Work out the finished part from the listing and answer in its coordinate system (mm). Round coordinates to 2 decimals unless told otherwise and drop trailing zeros. Write each loop counter-clockwise with the first axis right and the second up, starting at its lowest first coordinate (ties: lowest second). Pieces come first, ordered by that corner, then holes. Notation, with made-up numbers: M -16.75,-12.5 L -11.75,-12.5 A19 cw -11.75,-5.5 Z; hole C -15.5,45 d8. An arc over 180 degrees is marked long. One line per item, written item: value. Start each with the question number.
Q1. Find section B-B (x = 632). Write down the section's boundary in (y, z).
Q2. Find section A-A (y = 488.75). Write down the section's boundary in (x, z), and give its area (3 significant figures).
Q3. Consider probe 1 along X at (y, z) = (491.5, 1847); probe 2 along X at (y, z) = (486.5, 1922.5); probe 3 along Z at (x, y) = (610, 487.5). Determine where each line is inside the solid, lowest interval first.
Q4. Find section C-C (z = 1811). Write down the section's boundary in (x, y), and give its area (3 significant figures).
Q5. Given pin 1 Ø1 at (x, y) = (996.5, 487) entering from -Z; pin 2 Ø6.5 at (x, z) = (605.22, 1770.69) entering from +Y; pin 3 Ø2 at (y, z) = (486, 1840) entering from +X; pin 4 Ø6.5 at (x, z) = (979.33, 1620) entering from -Y, each flat-ended and moving along its own axis, determine where each tip first touches the part or whether it passes through.
from build123d import *

# Parameters (mm, degrees)
BOSS_EXTRUDE1_DEPTH                             = 12.7
CSK_FOR_M5_FLAT_HEAD_MACHINE_SCREW1_D           = 5.5
CSK_FOR_M5_FLAT_HEAD_MACHINE_SCREW1_DEPTH       = 12.7
CSK_FOR_M5_FLAT_HEAD_MACHINE_SCREW1_CSINK_D     = 10.4
CSK_FOR_M5_FLAT_HEAD_MACHINE_SCREW1_CSINK_ANGLE = 90


with BuildPart() as part:
    # Sketch1 → Boss-Extrude1 (new body)
    with BuildSketch(Plane(origin=(0, 484.313360873, 0), x_dir=(1, 0, 0), z_dir=(0, 1, 0))):
        Polygon((1096.723413016, -1803.339072227), (966.247715506, -1577.348534986), (705.296320486, -1577.348534986), (574.820622976, -1803.339072227), (705.296320486, -2029.329609468), (966.247715506, -2029.329609468), align=None)
    extrude(amount=BOSS_EXTRUDE1_DEPTH)

    # CSK for M5 Flat Head Machine Screw1
    with Locations(Plane(origin=(0, 497.013360873, 0), x_dir=(1, 0, 0), z_dir=(0, 1, 0))):
        with Locations((605.218725769, -1770.688013736), (692.218725769, -1619.999593477), (979.325310224, -1619.999593477), (1066.325310224, -1770.688013736), (748.77757228, -2019.323746494), (922.777572027, -2019.31436283)):
            CounterSinkHole(CSK_FOR_M5_FLAT_HEAD_MACHINE_SCREW1_D / 2, CSK_FOR_M5_FLAT_HEAD_MACHINE_SCREW1_CSINK_D / 2, depth=CSK_FOR_M5_FLAT_HEAD_MACHINE_SCREW1_DEPTH, counter_sink_angle=CSK_FOR_M5_FLAT_HEAD_MACHINE_SCREW1_CSINK_ANGLE)


solid = part.part
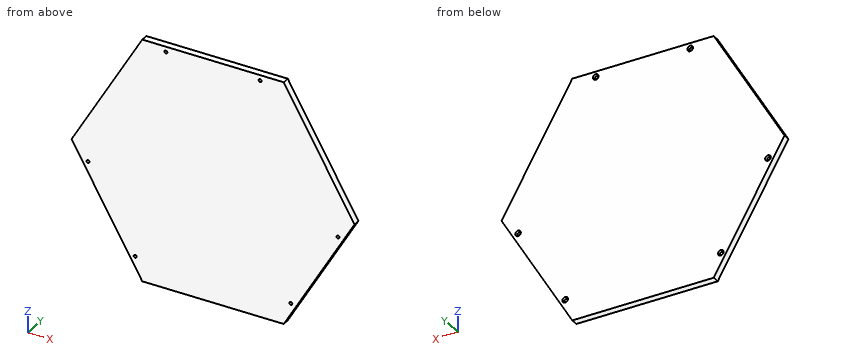
The answers:
1. outline: M 484.31,1704.3 L 497.01,1704.3 L 497.01,1902.38 L 484.31,1902.38 Z
2. outline: M 574.82,1803.34 L 705.3,1577.35 L 966.25,1577.35 L 1096.72,1803.34 L 966.25,2029.33 L 705.3,2029.33 Z; hole C 605.22,1770.69 d5.5; hole C 692.22,1620 d5.5; hole C 748.78,2019.32 d5.5; hole C 922.78,2019.31 d5.5; hole C 979.33,1620 d5.5; hole C 1066.33,1770.69 d5.5
2. area: 177,000 mm2
3. probe 1: 600.03 to 1071.52
3. probe 2: 643.62 to 1027.93
3. probe 3: 1742.41 to 1864.27
4. outline: M 579.24,484.31 L 1092.3,484.31 L 1092.3,497.01 L 579.24,497.01 Z
4. area: 6,520 mm2
5. pin 1: z = 1628.88
5. pin 2: y = 495.07
5. pin 3: x = 1076.13
5. pin 4: y = 484.31
